Build history of the part. All positions in model axes, mm. A direction names the side the tool comes from. Round coordinates to 2 decimals unless told otherwise and drop trailing zeros. Write each loop counter-clockwise with the first axis right and the second up, starting at its lowest first coordinate (ties: lowest second). Pieces come first, ordered by that corner, then holes.
Autodesk Inventor part; units mm, degrees
ref_plane "YZ Plane" through (0, 0, 0) normal (1, 0, 0) x (0, 1, 0)
ref_plane "XZ Plane" through (0, 0, 0) normal (0, 1, 0) x (-1, 0, 0)
ref_plane "XY Plane" through (0, 0, 0) normal (0, 0, 1) x (1, 0, 0)
sketch "Sketch1" plane through (0, 0, 0) normal (0, 0, 1) x (1, 0, 0)
  circle A0 centre (0, 0) radius 1.5
  circle A1 centre (10, 0) radius 1.5
  circle A2 centre (5, -10) radius 1.5
  line L0 (-10, 9) -> (20, 9)
  circle A3 centre (-4, -8) radius 1.5 construction
  circle A4 centre (-4, -18) radius 1.5 construction
  circle A5 centre (14, -8) radius 1.5 construction
  circle A6 centre (14, -18) radius 1.5 construction
  line L1 (-10, 9) -> (-10, -6)
  line L2 (-10, -6) -> (0, -6)
  line L3 (0, -6) -> (0, -15)
  line L4 (0, -15) -> (10, -15)
  line L5 (10, -15) -> (10, -6)
  line L6 (10, -6) -> (20, -6)
  line L7 (20, -6) -> (20, 9)
  dimension "d0" = 3
  dimension "d1" = 5
  dimension "d2" = 10
  dimension "d3" = 10
  dimension "d4" = 30
  dimension "d5" = 9
  dimension "d6" = 10
  dimension "d7" = 10
  dimension "d8" = 18
  dimension "d9" = 6
  dimension "d10" = 3
  dimension "d11" = 17
  dimension "d16" = 15
  dimension "d17" = 10
  dimension "d18" = 5
  dimension "d19" = 5
extrude "Extrusion1" add sketch "Sketch1" along normal blind 3
fillet "Fillet2" radius 4 6 edges at (0, -6, 1.5) (10, -6, 1.5) (10, -15, 1.5) (0, -15, 1.5) (-10, -6, 1.5) (20, -6, 1.5)
sketch "Sketch2" plane through (0, 0, 3) normal (0, 0, 1) x (1, 0, 0)
  line L0 (20, -2) -> (20, 9)
  line L1 (20, 9) -> (-10, 9)
  line L2 (-10, 9) -> (-10, -2)
  line L3 (-10, 5) -> (20, 5)
  dimension "d21" = 4
extrude "Extrusion2" add sketch "Sketch2" along normal blind 12
sketch "Sketch3" plane through (-10, 5, 3) normal (0, -1, 0) x (1, 0, 0)
  line L0 (0, 0) -> (0, 12)
  circle A0 centre (6, 6) radius 1.5
  circle A1 centre (24, 6) radius 1.5
  line L1 (0, -3) -> (30, -3)
  point P0 (10, -3)
  dimension "d24" = 18
  dimension "d25" = 6
  dimension "d26" = 9
  dimension "d27" = 3
extrude "Extrusion3" cut sketch "Sketch3" against normal up to next
sketch "Sketch4" plane through (-10, 5, 3) normal (0, -1, 0) x (1, 0, 0)
  circle A0 centre (6, 6) radius 1.5
  circle A1 centre (24, 6) radius 1.5
  line L0 (9.3486, 6) -> (7.6743, 3.1)
  line L1 (7.6743, 3.1) -> (4.3257, 3.1)
  line L2 (4.3257, 3.1) -> (2.6514, 6)
  line L3 (2.6514, 6) -> (4.3257, 8.9)
  line L4 (4.3257, 8.9) -> (7.6743, 8.9)
  line L5 (7.6743, 8.9) -> (9.3486, 6)
  circle A2 centre (24, 6) radius 1.5
  line L6 (27.3486, 6) -> (25.6743, 3.1)
  line L7 (25.6743, 3.1) -> (22.3257, 3.1)
  line L8 (22.3257, 3.1) -> (20.6514, 6)
  line L9 (20.6514, 6) -> (22.3257, 8.9)
  line L10 (22.3257, 8.9) -> (25.6743, 8.9)
  line L11 (25.6743, 8.9) -> (27.3486, 6)
  point P0 (10, -3)
  dimension "d30" = 5.8
extrude "Extrusion4" cut sketch "Sketch4" against normal blind 2.4
fillet "Fillet3" radius 3 1 edges at (5, 5, 3)
properties part number "ChimeraMountingBlock"
1) Wall check: L1, parallel to Z at x = -4, y = 7.9; L2, parallel to Y at x = 5, z = 1.15; L3, parallel to Y at x = 3.5, z = 13.5. Give the ranges that are in metal, low to high.
Results:
L1: z = 0 to 7.5, 10.5 to 15
L2: y = -15 to -11.5, -8.5 to 9
L3: y = 5 to 9
2) Pin check, flat tips, straight feed: pin 1 Ø5 at (x, y) = (0, 0) entering from -Z; pin 2 Ø6.5 at (x, z) = (-5, 8) entering from -Y; pin 3 Ø1 at (x, z) = (12, 11.5) entering from -Y; pin 4 Ø3.5 at (x, y) = (10, 0) entering from +Z. Stop position of each tip, or through.
Results:
pin 1: stops at z = 0
pin 2: stops at y = 4.73
pin 3: stops at y = 5
pin 4: stops at z = 3
3) Slice it at A-A (x = 5). Write the cut outline in (y, z), plus the area to 3 significant figures.
Results:
outline: (-15, 0) - (-11.5, 0) - (-11.5, 3) - (-15, 3) - close; (-8.5, 0) - (9, 0) - (9, 15) - (5, 15) - (5, 6) arc R3 cw to (2, 3) - (-8.5, 3) - close
area: 113 mm2
4) Which spindle directions (+Z, -Z, +X, -X, +Y, -Y) get a long thin tool onto all of the face, cutting with end or side? Do faces 4 (the flat face through (10, -10.5, 1.5)), 5 (the cylindrical face through (6.386, -9.425, 1.479)), 6 (the flat face through (5, 5, 10)), 7 (the flat face through (-1.5, 6.18, 10.47)), 8 (the flat face through (5, -15, 1)). Say none if no direction does.
Results:
face 4: +Z, -Z, +X, -Y
face 5: +Z, -Z
face 6: +Z, +X, -X, -Y
face 7: -Y
face 8: +Z, -Z, +X, -X, -Y
5) Mould opens along X. For faces 1 (the flat face through (5, -4, 3)), 2 (the cylindrical face through (8.797, -13.859, 1.521)), 3 (the flat face through (14, 6, 11.9)) say: released by +X, released by -X, zero draft, split by the parting line, or undercut.
Results:
face 1: zero draft
face 2: released by +X
face 3: undercut
6) Slice it at B-B (y = 7). Write the cut outline in (x, z).
Results:
outline: (-10, 0) - (20, 0) - (20, 15) - (-10, 15) - close; hole (-7.35, 9) - (-5.67, 6.1) - (-2.33, 6.1) - (-0.65, 9) - (-2.33, 11.9) - (-5.67, 11.9) - close; hole (10.65, 9) - (12.33, 6.1) - (15.67, 6.1) - (17.35, 9) - (15.67, 11.9) - (12.33, 11.9) - close
7) Slice it at C-C (z = 1). Write the cut outline in (x, y), plus the area to 3 significant figures.
Results:
outline: (-10, -2) arc R4 ccw to (-6, -6) - (-4, -6) arc R4 cw to (0, -10) - (0, -11) arc R4 ccw to (4, -15) - (6, -15) arc R4 ccw to (10, -11) - (10, -10) arc R4 cw to (14, -6) - (16, -6) arc R4 ccw to (20, -2) - (20, 9) - (-10, 9) - close; hole circle Ø3 at (0, 0); hole circle Ø3 at (5, -10); hole circle Ø3 at (10, 0)
area: 512 mm2
8) Slice it at D-D (z = 9.5). Write the cut outline in (x, y), plus the area to 3 significant figures.
Results:
outline: (-10, 5) - (-7.06, 5) - (-7.06, 7.4) - (-5.41, 7.4) - (-5.41, 9) - (-10, 9) - close; (-2.59, 7.4) - (-0.94, 7.4) - (-0.94, 5) - (10.94, 5) - (10.94, 7.4) - (12.59, 7.4) - (12.59, 9) - (-2.59, 9) - close; (15.41, 7.4) - (17.06, 7.4) - (17.06, 5) - (20, 5) - (20, 9) - (15.41, 9) - close
area: 81.6 mm2
